```python
from build123d import *

# Parameters (mm, degrees)
BOSS_EXTRUDE1_DEPTH = 15
SKETCH2_R           = 3
CUT_EXTRUDE1_DEPTH  = 10
SKETCH3_W           = 55.8
SKETCH3_H           = 21
CUT_EXTRUDE2_DEPTH  = 10
SKETCH4_R           = 6.9
SKETCH4_R_2         = 2
CUT_EXTRUDE3_DEPTH  = 5
CUT_EXTRUDE4_DEPTH  = 5
SKETCH7_R           = 3
CUT_EXTRUDE5_DEPTH  = 2
CUT_EXTRUDE6_DEPTH  = 3
SKETCH9_R           = 6.5
CUT_EXTRUDE7_DEPTH  = 3
SKETCH11_W          = 4
SKETCH11_H          = 12
BOSS_EXTRUDE2_DEPTH = 5
CUT_EXTRUDE9_DEPTH  = 4
SKETCH14_W          = 4
SKETCH14_H          = 12
BOSS_EXTRUDE3_DEPTH = 5
SKETCH15_W          = 3
SKETCH15_H          = 8
CUT_EXTRUDE10_DEPTH = 4
SKETCH16_R          = 1.5
CUT_EXTRUDE11_DEPTH = 7


with BuildPart() as part:
    # Sketch1 → Boss-Extrude1 (new body)
    with BuildSketch(Plane.XY):
        with BuildLine():
            Line((60, -15), (-60, -15))
            ThreePointArc((-60, -15), (-75, 0), (-60, 15))
            Line((-60, 15), (60, 15))
            ThreePointArc((60, 15), (75, 0), (60, -15))
        make_face()
    extrude(amount=BOSS_EXTRUDE1_DEPTH)

    # Sketch2 → Cut-Extrude1 (cut)
    with BuildSketch(Plane(origin=(0, 0, 0), x_dir=(-1, 0, 0), z_dir=(0, 0, -1))):
        with Locations((55, 0)):
            Circle(SKETCH2_R)
    extrude(amount=-CUT_EXTRUDE1_DEPTH, mode=Mode.SUBTRACT)

    # Sketch3 → Cut-Extrude2 (cut)
    with BuildSketch(Plane.XY.offset(15)):
        with Locations((34.58, 0.4)):
            Rectangle(SKETCH3_W, SKETCH3_H)
    extrude(amount=-CUT_EXTRUDE2_DEPTH, mode=Mode.SUBTRACT)

    # Sketch4 → Cut-Extrude3 (cut)
    with BuildSketch(Plane.XY.offset(5)):
        with Locations((45, 0)):
            Circle(SKETCH4_R)
        with Locations((58.98, -5.4)):
            Circle(SKETCH4_R_2)
        with Locations((58.98, 4.6)):
            Circle(SKETCH4_R_2)
        with Locations((10.18, 4.6)):
            Circle(SKETCH4_R_2)
        with Locations((10.18, -5.4)):
            Circle(SKETCH4_R_2)
    extrude(amount=-CUT_EXTRUDE3_DEPTH, mode=Mode.SUBTRACT)

    # Sketch6 → Cut-Extrude4 (cut)
    with BuildSketch(Plane.XY.offset(15)):
        with BuildLine():
            Line((-59.79767324, 3.94890295), (-12, 3.94890295))
            ThreePointArc((-12, 3.94890295), (-8.05109705, 0), (-12, -3.94890295))
            Line((-12, -3.94890295), (-59.79767324, -3.94890295))
            ThreePointArc((-59.79767324, -3.94890295), (-63.74657619, 0), (-59.79767324, 3.94890295))
        make_face()
    extrude(amount=-CUT_EXTRUDE4_DEPTH, mode=Mode.SUBTRACT)

    # Sketch7 → Cut-Extrude5 (cut)
    with BuildSketch(Plane(origin=(0, 0, 0), x_dir=(-1, 0, 0), z_dir=(0, 0, -1))):
        with Locations((-58.98, 4.6)):
            Circle(SKETCH7_R)
        with Locations((-58.98, -5.4)):
            Circle(SKETCH7_R)
        with Locations((-10.18, 4.6)):
            Circle(SKETCH7_R)
        with Locations((-10.18, -5.4)):
            Circle(SKETCH7_R)
    extrude(amount=-CUT_EXTRUDE5_DEPTH, mode=Mode.SUBTRACT)

    # Sketch8 → Cut-Extrude6 (cut)
    with BuildSketch(Plane(origin=(0, 0, 0), x_dir=(-1, 0, 0), z_dir=(0, 0, -1))):
        with BuildLine():
            Line((40, 4.65), (70, 4.65))
            ThreePointArc((70, 4.65), (74.65, 0), (70, -4.65))
            Line((70, -4.65), (40, -4.65))
            ThreePointArc((40, -4.65), (35.35, 0), (40, 4.65))
        make_face()
    extrude(amount=-CUT_EXTRUDE6_DEPTH, mode=Mode.SUBTRACT)

    # Sketch9 → Cut-Extrude7 (cut)
    with BuildSketch(Plane(origin=(0, 0, 0), x_dir=(-1, 0, 0), z_dir=(0, 0, -1))):
        with Locations((55, 0)):
            Circle(SKETCH9_R)
    extrude(amount=-CUT_EXTRUDE7_DEPTH, mode=Mode.SUBTRACT)

    # Sketch11 → Boss-Extrude2 (add)
    with BuildSketch(Plane.XY.offset(15)):
        Rectangle(SKETCH11_W, SKETCH11_H)
    extrude(amount=BOSS_EXTRUDE2_DEPTH)

    # Sketch13 → Cut-Extrude9 (cut)
    with BuildSketch(Plane(origin=(2, 0, 0), x_dir=(0, 0, -1), z_dir=(1, 0, 0))):
        Polygon((-15, 0), (-15, 4), (-18, 4), (-18, -4), (-15, -4), align=None)
    extrude(amount=-CUT_EXTRUDE9_DEPTH, mode=Mode.SUBTRACT)

    # Sketch14 → Boss-Extrude3 (add)
    with BuildSketch(Plane.XY.offset(15)):
        with Locations((-68, 0)):
            Rectangle(SKETCH14_W, SKETCH14_H)
    extrude(amount=BOSS_EXTRUDE3_DEPTH)

    # Sketch15 → Cut-Extrude10 (cut)
    with BuildSketch(Plane(origin=(-66, 0, 0), x_dir=(0, 0, -1), z_dir=(1, 0, 0))):
        with Locations((-16.5, 0)):
            Rectangle(SKETCH15_W, SKETCH15_H)
    extrude(amount=-CUT_EXTRUDE10_DEPTH, mode=Mode.SUBTRACT)

    # Sketch16 → Cut-Extrude11 (cut)
    with BuildSketch(Plane(origin=(0, 0, 3), x_dir=(-1, 0, 0), z_dir=(0, 0, -1))):
        with Locations((38.5, 0)):
            Circle(SKETCH16_R)
    extrude(amount=-CUT_EXTRUDE11_DEPTH, mode=Mode.SUBTRACT)


solid = part.part
```
Design review of the part built by this model. Coordinates are the model's own, in mm. A direction names the side the tool comes from. Give positions to 0.01 mm unless a question says otherwise; leave off trailing zeros. Write each loop counter-clockwise with the first axis right and the second up, starting at its lowest first coordinate (ties: lowest second). Pieces come first, ordered by that corner, then holes.
(1) Add section B-B (x = 10.18). Give the boundary of the cut face in (y, z).
Checked values:
outline: (-15, 0) - (-8.4, 0) - (-8.4, 2) - (-7.4, 2) - (-7.4, 5) - (-10.1, 5) - (-10.1, 15) - (-15, 15) - close; (-3.4, 2) - (-2.4, 2) - (-2.4, 0) - (1.6, 0) - (1.6, 2) - (2.6, 2) - (2.6, 5) - (-3.4, 5) - close; (6.6, 2) - (7.6, 2) - (7.6, 0) - (15, 0) - (15, 15) - (10.9, 15) - (10.9, 5) - (6.6, 5) - close
(2) Wall thickness on line 1 along Y through (x, z) = (10.18, 0.75); line 2 along Y through (x, z) = (58.98, 3.9); line 3 along X through (y, z) = (0.5, 18.5): over which ranges is each line inside the solid? List them lowest first.
Checked values:
line 1: y = -15 to -8.4, -2.4 to 1.6, 7.6 to 15
line 2: y = -15 to -7.4, -3.4 to 2.6, 6.6 to 15
line 3: x = -70 to -66, -2 to 2
(3) Add section C-C (y = 0). Give the number of separate pieces and of enclosed holes in the cut face, and give its area (3 significant figures).
Checked values:
separate pieces: 6
enclosed holes: 0
area: 1,180 mm2
(4) Tool access review of faces 4 (the face through (-36, 3.949, 13)), 5 (the face through (59, 7, 2)), 6 (the face through (-68, -6, 17)), 7 (the face through (-68, 6, 17)): name each direction out of +Z, -Z, +X, -X, +Y, -Y from which nothing blocks a thin tool from reaching the whole face with its end or side.
Checked values:
face 4: +Z
face 5: -Z
face 6: +Z, +X, -X, -Y
face 7: +Z, +X, -X, +Y
(5) Mouldability with a two-part tool opening along Z and no side actions: class faces 1 (the face through (-68, -4, 17)), 2 (the face through (34, 1, 5)), 3 (the face through (34, 10.9, 10)) as +Z half, -Z half, draft (parallel to the pull), parting line (faces both ways), or undercut.
Checked values:
face 1: undercut
face 2: +Z half
face 3: draft
(6) Add section D-D (x = -15). Give the boundary of the cut face in (y, z).
Checked values:
outline: (-15, 0) - (15, 0) - (15, 15) - (3.95, 15) - (3.95, 10) - (-3.95, 10) - (-3.95, 15) - (-15, 15) - close
(7) Clearance check with flat-ended pins moving along their axes: pin 1 Ø5 at (y, z) = (-6, 9) entering from -X; pin 2 Ø5 at (x, y) = (58.98, 4.6) entering from +Z; pin 3 Ø1 at (x, y) = (-7.5, -2.5) entering from +Z. State where each tip first meets the part, or that it passes through.
Checked values:
pin 1: stops at x = -74.59
pin 2: stops at z = 5
pin 3: stops at z = 15
(8) Add section A-A (x = -55). Give the boundary of the cut face in (y, z), and give its area (3 significant figures).
Checked values:
outline: (-15, 0) - (-6.5, 0) - (-6.5, 3) - (-3, 3) - (-3, 10) - (-3.95, 10) - (-3.95, 15) - (-15, 15) - close; (3, 3) - (6.5, 3) - (6.5, 0) - (15, 0) - (15, 15) - (3.95, 15) - (3.95, 10) - (3, 10) - close
area: 330 mm2
